Geometry check sheet. Reference: the model listing, model coordinates, mm. Face numbers are marked on the shaded views. A direction names the side the tool comes from. Give positions to 0.01 mm unless a question says otherwise; leave off trailing zeros. Order: outer loops, then holes, each group sorted by start corner. A loop starts at its lowest first (then second) coordinate and runs counter-clockwise, first axis right, second up. Notation, with made-up numbers: M 58.25,2.5 L 112.25,2.5 A20 cw 112.25,36.5 Z; hole C -14.75,-12.75 d5. An arc over 180 degrees is marked long. Put each result on its own line as item: value. Start each with the question number.
Q1. Access from +Z, -Z, +X, -X, +Y, -Y to the whole of each face (thin tool, end or side, straight path). Record for the marked faces 4, 5 and 6.
Q2. Section check D-D on x = 15. Record the cut outline in (y, z), then the cut area to 3 significant figures.
Q3. Section check B-B on x = 30. Record the cut outline in (y, z), then the cut area to 3 significant figures.
Q4. Go/stop test with flat-tipped pins: pin 1 (6 mm diameter, centred on x = 30.5, y = -3, fed in from +Z); pin 2 (2 mm diameter, centred on x = 25.5, z = 4.5, fed in from -Y); pin 3 (3 mm diameter, centred on x = 31.5, z = -3.5, fed in from +Y). Record where each tip stops, or that it passes through.
Q5. Section check C-C on y = 23.5. Record the cut outline in (x, z), then the cut area to 3 significant figures.
Q6. Section check A-A on z = 11.5. Record the cut outline in (x, y).
Q7. Mould release check, pull along Y, two halves, no side actions. Record for the marked faces 1, 2 and 3: +Y half, -Y half, draft (parallel to the pull), parting line (faces both ways), or undercut.
Q8. Material ranges on L1, parallel to Z at x = 20, y = 19; L2, parallel to Z at x = 30.5, y = 16.5; L3, parallel to Y at x = 30, z = -10, recorded low to high.
Autodesk Inventor part; units mm, degrees
ref_plane "YZ Plane" through (0, 0, 0) normal (1, 0, 0) x (0, 1, 0)
ref_plane "XZ Plane" through (0, 0, 0) normal (0, 1, 0) x (-1, 0, 0)
ref_plane "XY Plane" through (0, 0, 0) normal (0, 0, 1) x (1, 0, 0)
sketch "Szkic1" plane through (0, 0, 0) normal (1, 0, 0) x (0, 1, 0)
  line L0 (28.1466, 19.5) -> (-31.8534, 19.5)
  line L1 (-31.8534, 19.5) -> (-31.8534, -19.5)
  line L2 (-31.8534, -19.5) -> (28.1466, -19.5)
  line L3 (28.1466, -19.5) -> (28.1466, 19.5)
  line L4 (28.1466, 0) -> (28.1466, 5.5)
  line L5 (28.1466, 5.5) -> (6.1466, 5.5)
  line L6 (6.1466, 5.5) -> (6.1466, 0)
  line L7 (28.1466, -5.5) -> (6.1466, -5.5)
  line L8 (6.1466, -5.5) -> (6.1466, 0)
  line L9 (18.1466, 12.5) -> (6.1466, 12.5)
  line L10 (6.1466, 12.5) -> (6.1466, -12.5)
  line L11 (6.1466, -12.5) -> (18.1466, -12.5)
  line L12 (18.1466, -12.5) -> (18.1466, 12.5)
  line L13 (-31.8534, 9.5) -> (-27.8534, 9.5)
  line L14 (-27.8534, 9.5) -> (-18.3534, 0)
  line L15 (-31.8534, 0) -> (0, 0)
  line L16 (-31.8534, -9.5) -> (-27.8534, -9.5)
  line L17 (-27.8534, -9.5) -> (-18.3534, 0)
  point P0 (12.1466, 0)
  point P1 (6.1466, 2.75)
  point P2 (18.1466, -5.5)
  point P3 (6.1466, -5.5)
  point P4 (18.1466, 5.5)
  dimension "d0" = 60
  dimension "d1" = 39
  dimension "d2" = 22
  dimension "d4" = 12
  dimension "d5" = 25
  dimension "d6" = 135
  dimension "d7" = 10
  dimension "d8" = 4
  dimension "d9" = 9.5
extrude "Wyciągnięcie proste1" add sketch "Szkic1" along normal blind 60 contours L3 L5 L12 L9 L10 L6 L8 L11 L7 L2 L1 L16 L17 L14 L13 L0
sketch "Szkic2" plane through (0, -31.8534, 19.5) normal (0, 0, 1) x (1, 0, 0)
  point P0 (0, 31.8534)
  point P1 (30, 30)
hole "Otwór1" at (30, -1.8534, 19.5) direction (0, 0, -1) diameter 8 end through all counterbore diameter 12 counterbore depth 4
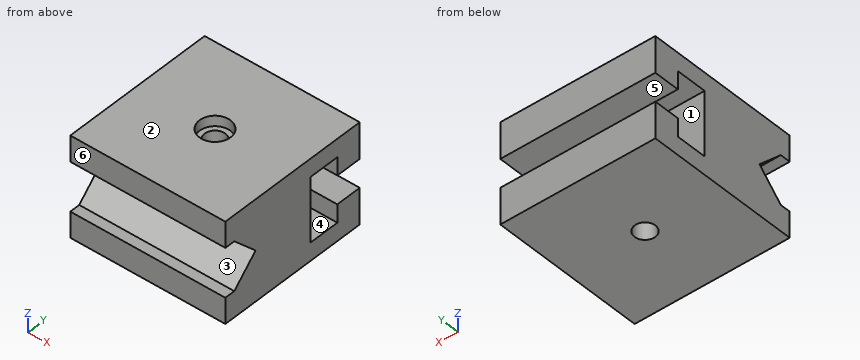
Results found:
1. face 4: +X, -X
1. face 5: +X, -X, +Y
1. face 6: +Z, -Z, +X, -X, -Y
2. outline: M -31.85,-19.5 L 28.15,-19.5 L 28.15,-5.5 L 18.15,-5.5 L 18.15,-12.5 L 6.15,-12.5 L 6.15,12.5 L 18.15,12.5 L 18.15,5.5 L 28.15,5.5 L 28.15,19.5 L -31.85,19.5 L -31.85,9.5 L -27.85,9.5 L -18.35,0 L -27.85,-9.5 L -31.85,-9.5 Z
2. area: 1,760 mm^2
3. outline: M -31.85,-19.5 L -5.85,-19.5 L -5.85,15.5 L -7.85,15.5 L -7.85,19.5 L -31.85,19.5 L -31.85,9.5 L -27.85,9.5 L -18.35,0 L -27.85,-9.5 L -31.85,-9.5 Z; M 2.15,-19.5 L 28.15,-19.5 L 28.15,-5.5 L 18.15,-5.5 L 18.15,-12.5 L 6.15,-12.5 L 6.15,12.5 L 18.15,12.5 L 18.15,5.5 L 28.15,5.5 L 28.15,19.5 L 4.15,19.5 L 4.15,15.5 L 2.15,15.5 Z
3. area: 1,440 mm^2
4. pin 1: stops at z = 15.5
4. pin 2: stops at y = -23.85
4. pin 3: stops at y = 6.15
5. outline: M 0,-19.5 L 60,-19.5 L 60,-5.5 L 0,-5.5 Z; M 0,5.5 L 60,5.5 L 60,19.5 L 0,19.5 Z
5. area: 1,680 mm^2
6. outline: M 0,-31.85 L 60,-31.85 L 60,6.15 L 0,6.15 Z; M 0,18.15 L 60,18.15 L 60,28.15 L 0,28.15 Z; hole C 30,-1.85 d8
7. face 1: undercut
7. face 2: draft
7. face 3: -Y half
8. L1: z = -19.5 to -5.5, 5.5 to 19.5
8. L2: z = -19.5 to -12.5, 12.5 to 19.5
8. L3: y = -31.85 to -5.85, 2.15 to 6.15, 18.15 to 28.15
